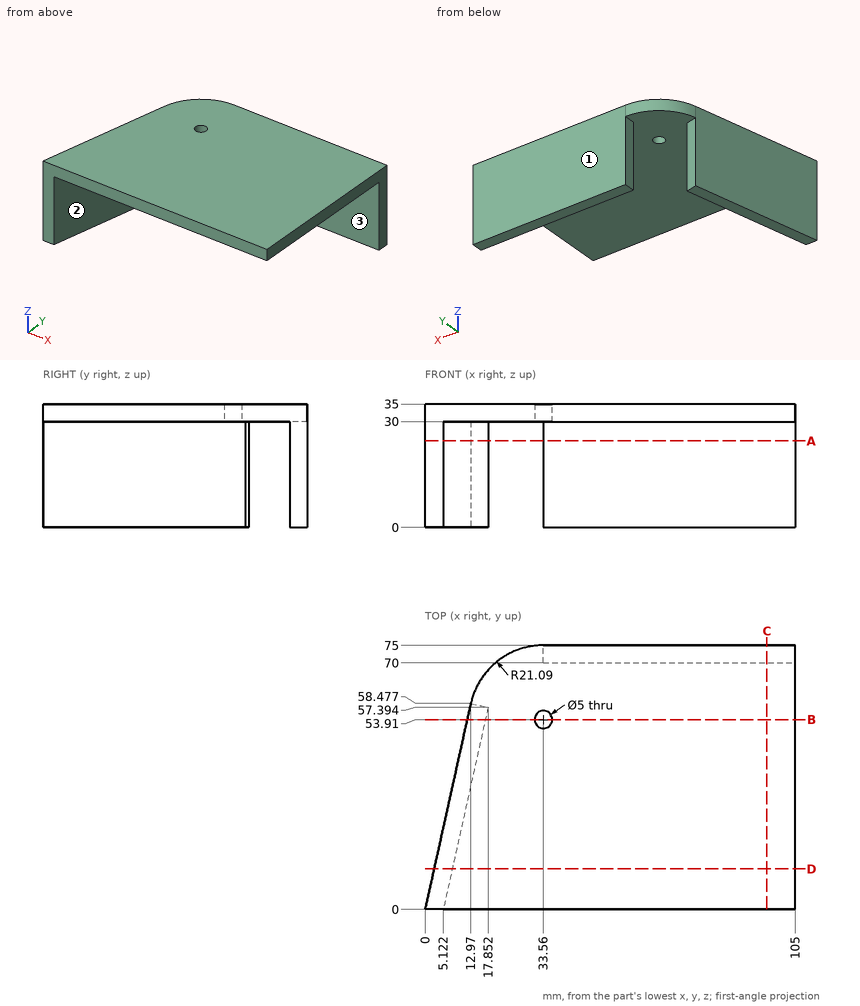
Answer from the drawing. Dimensions are ordinates in mm from the lowest x, y and z of the part. A direction names the side the tool comes from. Round coordinates to 2 decimals unless told otherwise and drop trailing zeros. Order: outer loops, then holes, each group sorted by start corner. A loop starts at its lowest first (then second) coordinate and runs counter-clockwise, first axis right, second up. Notation, with made-up numbers: (-36, 1) - (9, 1) arc R13 ccw to (9, 25) - close; hole circle Ø4 at (18.5, -3). An arc over 180 degrees is marked (long way). Put each result on its own line as item: value. Start each with the question number.
(1) Given P1, Ø12, axis at x = 38.5, z = 13.5, coming from the -Y side; P2, Ø3, axis at x = 56.5, y = 9.5, coming from the -Z side; P3, Ø8, axis at y = 53, z = 19.5, coming from the +X side (1 decimal), each flat-ended and moving along its own axis, determine where each tip first touches the part or whether it passes through.
(2) Straight lines are drawn through the part: probe 1 along Y at (x, z) = (33.56, 32.8); probe 2 along Y at (x, z) = (36.5, 10); probe 3 along X at (y, z) = (53, 32) (1 decimal). For each, find the intervals that lie inside material, in ascending order. Write a range as from..to.
(3) Find section B-B (y = 53.91). Give the vertices of the cut face in (x, z).
(4) Find section A-A (z = 24.5). Give the vertices of the cut face in (x, y) (1 decimal), plus the area to 3 significant figures.
(5) Find section C-C (x = 97). Give the vertices of the cut face in (y, z).
(6) For the marked faces 1, 2 and 3, determine the directions among +Z, -Z, +X, -X, +Y, -Y from which every point of the face is accessible in a straight line to the end or side of a thin tool.
(7) Find section D-D (y = 11.5). Give the vertices of the cut face in (x, z).
Reply:
1. P1: y = 70
1. P2: z = 30
1. P3: x = 17.8
2. probe 1: 0..51.41, 56.41..75
2. probe 2: 70..75
2. probe 3: 11.8..31.2, 35.9..105
3. outline: (11.96, 0) - (17.08, 0) - (17.08, 30) - (31.06, 30) - (31.06, 35) - (11.96, 35) - close; (36.06, 30) - (105, 30) - (105, 35) - (36.06, 35) - close
4. outline: (0, 0) - (5.1, 0) - (17.9, 57.4) - (13, 58.5) - close; (33.6, 70) - (105, 70) - (105, 75) - (33.6, 75) - close
4. area: 654 mm^2
5. outline: (0, 30) - (70, 30) - (70, 0) - (75, 0) - (75, 35) - (0, 35) - close
6. face 1: +Z, -Z, +X, -X, +Y
6. face 2: -Z, +X, -Y
6. face 3: -Z, +X, -X, -Y
7. outline: (2.55, 0) - (7.67, 0) - (7.67, 30) - (105, 30) - (105, 35) - (2.55, 35) - close
